```python
from build123d import *

# Parameters (mm, degrees)
F0_W     = 300
F0_H     = 300
F1_DEPTH = 30
F2_W     = 260.52019
F2_H     = 271.989614
F3_DEPTH = 25
F5_DEPTH = 25


with BuildPart() as f1:
    # F0 (on Front) → F1 (new body)
    with BuildSketch(Plane.XZ):
        Rectangle(F0_W, F0_H)
    extrude(amount=F1_DEPTH)

    # F2 (on face) → F3 (cut)
    with BuildSketch(Plane.XZ.offset(30)):
        Rectangle(F2_W, F2_H)
    extrude(amount=-F3_DEPTH, mode=Mode.SUBTRACT)

    # F4 (on face) → F5 (join)
    with BuildSketch(Plane.XZ.offset(5)):
        with BuildLine():
            ThreePointArc((-45.873974, -38.844235), (-69.621389, -56.0838), (-40.916645, -49.986262))
            ThreePointArc((-40.916645, -49.986262), (-42.2119, -43.888724), (-45.873974, -38.844235))
        make_face()
        with BuildLine():
            ThreePointArc((16.034492, 24.293919), (9.001979, 28.862168), (7.686935, 20.57991))
            ThreePointArc((7.686935, 20.57991), (13.067005, 19.725671), (16.034492, 24.293919))
        make_face()
    extrude(amount=F5_DEPTH)


solid = f1.part
```
Model file for the job. Use its own axes, mm. A direction names the side the tool comes from. Give positions to 0.01 mm unless a question says otherwise; leave off trailing zeros. Loops run counter-clockwise (first coordinate to the right, second up) from the corner with the lowest first, then second, coordinate; pieces in that order, holes last. Notation, with made-up numbers: (-32.75, -36.5) - (-28.75, -36.5) arc R18 cw to (-28.75, -13.5) - close; hole circle Ø4 at (48, -3.5). An arc over 180 degrees is marked (long way). One line per item, written item: value. Start each with the question number.
1. Pull direction Z, two halves, no side cores. Call faces 1 (the flat face through (-2, -5, 2)), 2 (the flat face through (-2, -15, 150)), 3 (the flat face through (-2, 0, 2)), 4 (the flat face through (-2, -15, -150)): pulls with the +Z half, pulls with the -Z half, needs draft (parallel to the pull), parting line crosses it, or undercut.
2. Slice it at D-D (z = -58.5). List the corners of the cut face in (x, y).
3. Slice it at A-A (y = -26.5). List the corners of the cut face in (x, z), plus the area to 3 significant figures.
4. Probe L1, parallel to Z at x = -110.5, y = -20.75; L2, parallel to X at y = -24.25, z = 88; L3, parallel to Z at x = -67.5, y = -19. List the from-to ranges inside material, lowest first. Write a range as from..to.
5. Slice it at B-B (z = 1). List the corners of the cut face in (x, y), plus the area to 3 significant figures.
6. Slice it at C-C (x = 100.5). List the corners of the cut face in (y, z), plus the area to 3 significant figures.
7. Pin check, flat tips, straight feed: pin 1 (1.5 mm diameter, centred on x = -35.5, z = -31, fed in from -Y); pin 2 (8 mm diameter, centred on x = 52.5, z = 87.5, fed in from +Y). Stop position of each tip, or through.
8. Which spindle directions (+Z, -Z, +X, -X, +Y, -Y) get a long thin tool onto all of the face, cutting with end or side? Do faces 5 (the flat face through (150, -15, -2)), 6 (the flat face through (-2, -18, -135.995)). Say none if no direction does.
Solution:
1. face 1: undercut
1. face 2: pulls with the +Z half
1. face 3: needs draft
1. face 4: pulls with the -Z half
2. outline: (-150, -30) - (-130.26, -30) - (-130.26, -5) - (-68.27, -5) - (-68.27, -30) - (-43.57, -30) - (-43.57, -5) - (130.26, -5) - (130.26, -30) - (150, -30) - (150, 0) - (-150, 0) - close
3. outline: (-150, -150) - (150, -150) - (150, 150) - (-150, 150) - close; circle Ø30 at (-55.92, -49.99); circle Ø10 at (11.03, 24.29); hole (-130.26, -135.99) - (130.26, -135.99) - (130.26, 135.99) - (-130.26, 135.99) - close
3. area: 19,900 mm^2
4. L1: z = -150..-135.99, 135.99..150
4. L2: x = -150..-130.26, 130.26..150
4. L3: z = -150..-135.99, -59.52..-40.46, 135.99..150
5. outline: (-150, -30) - (-130.26, -30) - (-130.26, -5) - (130.26, -5) - (130.26, -30) - (150, -30) - (150, 0) - (-150, 0) - close
5. area: 2,490 mm^2
6. outline: (-30, -150) - (0, -150) - (0, 150) - (-30, 150) - (-30, 135.99) - (-5, 135.99) - (-5, -135.99) - (-30, -135.99) - close
6. area: 2,200 mm^2
7. pin 1: stops at y = -5
7. pin 2: stops at y = 0
8. face 5: +Z, -Z, +X, +Y, -Y
8. face 6: -Y
